Verification items for the finished model (mm, model axes). Face numbers are marked on the shaded views. A direction names the side the tool comes from. Give positions to 0.01 mm unless a question says otherwise; leave off trailing zeros. Order: outer loops, then holes, each group sorted by start corner. A loop starts at its lowest first (then second) coordinate and runs counter-clockwise, first axis right, second up.
(1) Scan lines: L1, parallel to X at y = -26, z = 26.5; L2, parallel to Z at x = -10, y = 23; L3, parallel to Y at x = 0, z = 7.4. Record each from-to range of solid material in increasing order.
(2) Sectioned sample at C-C on z = 12.5. Record the cut outline in (x, y), plus the area to 3 significant figures.
(3) Gauge pin test, flat ends, axial feed: pin 1 (15 mm diameter, centred on x = 6.5, y = 10, fed in from +Z); pin 2 (3.5 mm diameter, centred on x = 24.75, y = 24.75, fed in from +Z); pin 3 (1 mm diameter, centred on x = -8.5, z = 18, fed in from +Y). Record the tip position at first contact, or that the pin passes through.
(4) Sectioned sample at D-D on y = -3.5. Record the cut outline in (x, z).
(5) Sectioned sample at B-B on y = 9. Record the cut outline in (x, z).
(6) Sectioned sample at A-A on x = 0. Record the cut outline in (y, z), plus the area to 3 significant figures.
(7) Mould release check, pull along Y, two halves, no side actions. Record for the marked faces 5, 6 and 7: pulls with the +Y half, pulls with the -Y half, needs draft (parallel to the pull), parting line crosses it, or undercut.
(8) Access from +Z, -Z, +X, -X, +Y, -Y to the whole of each face (thin tool, end or side, straight path). Record for the marked faces 1, 2, 3 and 4.
```python
from build123d import *

# Parameters (mm, degrees)
SKETCH_1_R               = 19
EXTRUDE_1_DEPTH          = 31.5
SKETCH_2_R               = 25
CUT_EXTRUDE_1_DEPTH      = 10
PATTERN_CIRCULAR_1_COUNT = 4
SKETCH_6_R               = 19
SKETCH_6_R_2             = 16
EXTRUDE_2_DEPTH          = 8
SKETCH_7_R               = 20
CUT_EXTRUDE_2_DEPTH      = 1.5
SKETCH_9_R               = 4
CUT_EXTRUDE_3_DEPTH      = 20
PATTERN_CIRCULAR_2_COUNT = 4


with BuildPart() as part:
    # 草图1 → 凸台-拉伸1 (new body)
    with BuildSketch(Plane.XY):
        Polygon((30, 26), (26, 30), (-26, 30), (-30, 26), (-30, -26), (-26, -30), (26, -30), (30, -26), align=None)
        Circle(SKETCH_1_R, mode=Mode.SUBTRACT)
    extrude(amount=EXTRUDE_1_DEPTH)

    # 草图2 → 切除-拉伸1 (cut)
    with BuildSketch(Plane.XY.offset(31.5)):
        Circle(SKETCH_2_R)
    extrude(amount=-CUT_EXTRUDE_1_DEPTH, mode=Mode.SUBTRACT)

    # 草图4 → M5 螺纹孔1 (revolve, cut)
    with BuildSketch(Plane(origin=(24.748737342, 24.748737342, 31.5), x_dir=(0, -1, 0), z_dir=(1, 0, 0))):
        Polygon((0, 0), (0, 15.2618073), (2.1, 14), (2.1, 0), align=None)
    hole_wizard_m5_1 = revolve(axis=Axis((24.748737342, 24.748737342, 37.85), (0, 0, -1)), mode=Mode.SUBTRACT)

    # 阵列(圆周)1: M5 螺纹孔1 ×4 about axis
    pattern_circular_1_axis = Axis((0, 0, 0), (0, 0, 1))
    for i in range(1, PATTERN_CIRCULAR_1_COUNT):
        add(hole_wizard_m5_1.rotate(pattern_circular_1_axis, i * 360 / PATTERN_CIRCULAR_1_COUNT), mode=Mode.SUBTRACT)

    # 草图6 → 凸台-拉伸2 (add)
    with BuildSketch(Plane(origin=(0, 0, 0), x_dir=(-1, 0, 0), z_dir=(0, 0, -1))):
        Circle(SKETCH_6_R)
        Circle(SKETCH_6_R_2, mode=Mode.SUBTRACT)
    extrude(amount=-EXTRUDE_2_DEPTH)

    # 草图7 → 切除-拉伸2 (cut)
    with BuildSketch(Plane.XY.offset(8)):
        Circle(SKETCH_7_R)
    extrude(amount=-CUT_EXTRUDE_2_DEPTH, mode=Mode.SUBTRACT)

    # 草图9 → 切除-拉伸3 (cut)
    with BuildSketch(Plane(origin=(0, 30, 0), x_dir=(1, 0, 0), z_dir=(0, 1, 0))):
        with Locations(Location((-10, -15.5, 0), (0, 0, 270))):
            Circle(SKETCH_9_R)
    cut_extrude_3 = extrude(amount=-CUT_EXTRUDE_3_DEPTH, mode=Mode.SUBTRACT)

    # 阵列(圆周)2: 切除-拉伸3 ×4 about axis
    pattern_circular_2_axis = Axis((0, 0, 31.5), (0, 0, -1))
    for i in range(1, PATTERN_CIRCULAR_2_COUNT):
        add(cut_extrude_3.rotate(pattern_circular_2_axis, i * 360 / PATTERN_CIRCULAR_2_COUNT), mode=Mode.SUBTRACT)


solid = part.part
```
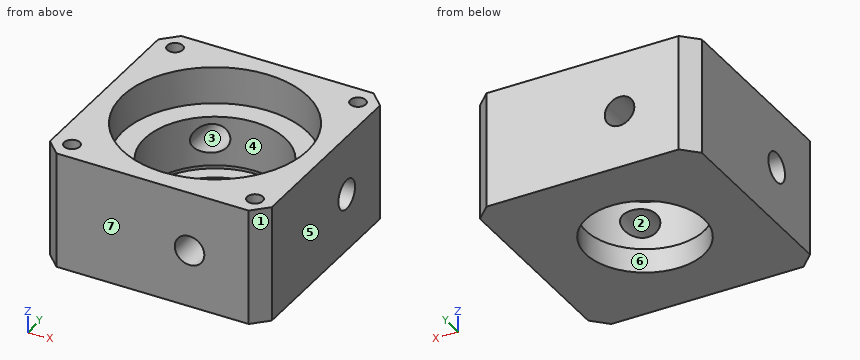
Ans:
1. L1: x = -30 to -26.44, -23.06 to 23.06, 26.44 to 30
1. L2: z = 0 to 11.5, 19.5 to 31.5
1. L3: y = -30 to -20, 20 to 30
2. outline: (-30, -26) - (-26, -30) - (7.35, -30) - (7.35, -17.52) arc R19 cw to (-14.18, -12.65) - (-30, -12.65) - close; (-30, -7.35) - (-17.52, -7.35) arc R19 cw to (-12.65, 14.18) - (-12.65, 30) - (-26, 30) - (-30, 26) - close; (-7.35, 17.52) arc R19 cw to (14.18, 12.65) - (30, 12.65) - (30, 26) - (26, 30) - (-7.35, 30) - close; (12.65, -30) - (26, -30) - (30, -26) - (30, 7.35) - (17.52, 7.35) arc R19 cw to (12.65, -14.18) - close
2. area: 2,140 mm2
3. pin 1: stops at z = 21.5
3. pin 2: stops at z = 17.29
3. pin 3: stops at y = -16.73
4. outline: (-30, 0) - (-15.61, 0) - (-15.61, 6.5) - (-19.69, 6.5) - (-19.69, 8) - (-18.67, 8) - (-18.67, 21.5) - (-24.75, 21.5) - (-24.75, 31.5) - (-30, 31.5) - close; (15.61, 0) - (30, 0) - (30, 31.5) - (24.75, 31.5) - (24.75, 21.5) - (18.67, 21.5) - (18.67, 8) - (19.69, 8) - (19.69, 6.5) - (15.61, 6.5) - close
5. outline: (-30, 0) - (-13.23, 0) - (-13.23, 6.5) - (-17.86, 6.5) - (-17.86, 8) - (-16.73, 8) - (-16.73, 21.5) - (-23.32, 21.5) - (-23.32, 31.5) - (-30, 31.5) - close; (13.23, 0) - (30, 0) - (30, 11.63) - (16.73, 11.63) - (16.73, 8) - (17.86, 8) - (17.86, 6.5) - (13.23, 6.5) - close; (16.73, 19.37) - (30, 19.37) - (30, 31.5) - (23.32, 31.5) - (23.32, 21.5) - (16.73, 21.5) - close
6. outline: (-30, 0) - (-16, 0) - (-16, 6.5) - (-20, 6.5) - (-20, 8) - (-19, 8) - (-19, 21.5) - (-25, 21.5) - (-25, 31.5) - (-30, 31.5) - close; (16, 0) - (30, 0) - (30, 31.5) - (25, 31.5) - (25, 21.5) - (19, 21.5) - (19, 8) - (20, 8) - (20, 6.5) - (16, 6.5) - close
6. area: 609 mm2
7. face 5: needs draft
7. face 6: undercut
7. face 7: pulls with the -Y half
8. face 1: +Z, -Z, +X, -Y
8. face 2: -Y
8. face 3: +Y
8. face 4: +Z
